CAD build for the part. Positions are in the model's coordinates, mm. A direction names the side the tool comes from. Round coordinates to 2 decimals unless told otherwise and drop trailing zeros. Order: outer loops, then holes, each group sorted by start corner. A loop starts at its lowest first (then second) coordinate and runs counter-clockwise, first axis right, second up.
Autodesk Inventor part; units mm, degrees
ref_plane "YZ Plane" through (0, 0, 0) normal (1, 0, 0) x (0, 1, 0)
ref_plane "XZ Plane" through (0, 0, 0) normal (0, 1, 0) x (-1, 0, 0)
ref_plane "XY Plane" through (0, 0, 0) normal (0, 0, 1) x (1, 0, 0)
sketch "Sketch1" plane through (0, 0, 0) normal (0, 0, 1) x (1, 0, 0)
  line L0 (-24.7628, 24.1619) -> (95.2372, 24.1619)
  line L1 (95.2372, 24.1619) -> (95.2372, -75.8381)
  line L2 (95.2372, -75.8381) -> (-24.7628, -75.8381)
  line L3 (-24.7628, -75.8381) -> (-24.7628, 24.1619)
  point P0 (0, 0)
  dimension "d0" = 120
  dimension "d1" = 100
extrude "Extrusion1" add sketch "Sketch1" along normal blind 80
sketch "Sketch2" plane through (-24.7628, -75.8381, 0) normal (-1, 0, 0) x (0, 0, 1)
  line L0 (0, 0) -> (80, 0)
  line L1 (4.914, 93.7072) -> (77, 93.7072)
  line L2 (77, 93.7072) -> (77, 0)
  line L3 (77, 0) -> (4.914, 0)
  line L4 (4.914, 0) -> (4.914, 93.7072)
  line L5 (80, 100) -> (80, 0)
  line L6 (0, 100) -> (0, 0)
  point P0 (0, 75.8381)
  point P1 (4.914, 0)
  dimension "d6" = 3
  dimension "d108" = 4.914
extrude "Extrusion2" cut sketch "Sketch2" against normal blind 60
sketch "Sketch3" plane through (-24.7628, 24.1619, 0) normal (0, 1, 0) x (1, 0, 0)
  line L0 (0, 0) -> (0, -4.914)
  line L1 (0, 0) -> (0, -31.38)
  circle A0 centre (26.718, -35) radius 11
  line L2 (120, 0) -> (0, 0)
  point P0 (24.7628, 0)
  dimension "d7" = 31.38
  dimension "d9" = 22
  dimension "d109" = 35
extrude "Extrusion3" cut sketch "Sketch3" against normal blind 80
sketch "Sketch8" plane through (0, 0, 0) normal (0, 0, -1) x (-1, 0, 0)
  line L0 (-95.2372, 24.1619) -> (24.7628, 24.1619)
  line L1 (-1.9784, 24.1619) -> (-38.1484, 24.1619)
  circle A0 centre (-1.7434, -26.1683) radius 3.5
  circle A1 centre (-10.4934, -46.1683) radius 1.575
  circle A2 centre (7.0066, -46.1683) radius 1.575
  line L2 (7.0066, -46.1683) -> (-10.4934, -46.1683)
  line L3 (-1.7434, -26.1683) -> (-1.7434, -46.1683)
  point P0 (0, 0)
  point P1 (-4.8068, -28.0128)
  dimension "d26" = 36.17
  dimension "d143" = 3.15
  dimension "d144" = 3.15
  dimension "d145" = 20
sketch "Sketch9" plane through (0, 0, 80) normal (0, 0, 1) x (1, 0, 0)
  line L0 (95.2372, 24.1619) -> (-24.7628, 24.1619)
  line L1 (41.408, 24.1619) -> (95.2372, 24.1619)
  line L2 (95.2372, 24.1619) -> (95.2372, -75.6591)
  line L3 (95.2372, -75.6591) -> (41.408, -75.6591)
  line L4 (41.408, -75.6591) -> (41.408, 24.1619)
  point P0 (0, 0)
extrude "Extrusion8" cut sketch "Sketch9" against normal blind 82.75
sketch "Sketch11" plane through (41.408, -75.6591, 80) normal (0, 1, 0) x (1, 0, 0)
  line L0 (0, 0) -> (-66.1708, 0)
  line L1 (-66.1708, 80) -> (53.8292, 80)
  line L2 (0, 0) -> (53.8292, 0)
  line L3 (53.8292, 0) -> (53.8292, 80)
  line L4 (53.8292, 80) -> (0, 80)
  line L5 (0, 80) -> (0, 0)
  point P0 (-41.408, 80)
extrude "Extrusion9" cut sketch "Sketch11" against normal blind 82.75
sketch "Sketch16" plane through (-24.7628, -75.8381, 77) normal (0, -1, 0) x (1, 0, 0)
  line L0 (0, -72.086) -> (0, 0)
  line L1 (0, 0) -> (60, 0)
  line L2 (0, -72.086) -> (60, -72.086)
  line L3 (60, -72.086) -> (60, 0)
  line L4 (60, 0) -> (0, 0)
  line L5 (0, 0) -> (0, -72.086)
  circle A0 centre (26.718, -42) radius 11
  circle A1 centre (26.718, -42) radius 5
  point P0 (24.7628, -77)
extrude "Extrusion14" add sketch "Sketch16" against normal blind 10 contours L0 L1 L3 L2
ref_plane "Work Plane1" through (-34.7628, -75.8381, 80) normal (-1, 0, 0) x (0, 0, 1)
sketch "Sketch24" plane through (-34.7628, -75.8381, 80) normal (-1, 0, 0) x (0, 0, 1)
  line L0 (-131.9676, 100) -> (-77.9351, 100)
  line L1 (-77.9351, 100) -> (-77.9351, -1.253)
  line L2 (-77.9351, -1.253) -> (-131.9676, -1.253)
  line L3 (-131.9676, -1.253) -> (-131.9676, 100)
  point P0 (-80, 75.8381)
extrude "Extrusion19" cut sketch "Sketch24" against normal blind 103.25
sketch "Sketch27" plane through (0, 0, 80) normal (0, 0, 1) x (1, 0, 0)
  line L0 (-24.7628, -75.8381) -> (41.408, -75.8381)
  circle A0 centre (15.3226, -32.8381) radius 1.5
  line L1 (15.3226, -32.8381) -> (1.3226, -32.8381)
  line L2 (15.3226, -35.3779) -> (15.3226, -32.8381)
  circle A1 centre (15.3226, -27.8381) radius 1.5
  circle A2 centre (1.3226, -32.8381) radius 1.5
  circle A3 centre (1.3226, -27.8381) radius 1.5
  line L3 (41.408, 24.1619) -> (-24.7628, 24.1619)
  point P0 (0, 0)
  dimension "d125" = 5
  dimension "d128" = 14
  dimension "d169" = 52
extrude "Extrusion22" cut sketch "Sketch27" against normal blind 20
extrude "Extrusion24" cut sketch "Sketch8" against normal blind 10
sketch "Sketch28" plane through (41.408, 24.1619, 2.0649) normal (0, 0, -1) x (-1, 0, 0)
  line L0 (0, -100) -> (0, 0)
  line L1 (66.1708, -90) -> (66.1708, -6.2928)
  line L2 (0, 0) -> (66.1708, 0)
  line L3 (66.1708, 0) -> (66.1708, -12.3951)
  line L4 (66.1708, -12.3951) -> (0, -12.3951)
  line L5 (0, -12.3951) -> (0, 0)
  point P0 (41.408, -24.1619)
  point P1 (0, -12.3951)
extrude "Extrusion25" add sketch "Sketch28" along normal blind 80
sketch "Sketch29" plane through (-24.7628, 11.7668, 2.0649) normal (0, -1, 0) x (1, 0, 0)
  line L0 (66.1708, -80) -> (0, -80)
  line L1 (66.1708, -80) -> (66.1708, -78.32)
  line L2 (66.1708, 0) -> (66.1708, -80)
  circle A0 centre (56.4908, -78.32) radius 0.75
  line L3 (56.4908, -78.32) -> (13.4908, -78.32)
  line L4 (56.4908, -61.93) -> (56.4908, -78.32)
  circle A1 centre (13.4908, -78.32) radius 0.75
  circle A2 centre (56.4908, -60.32) radius 0.75
  circle A3 centre (13.4908, -60.32) radius 0.75
  point P0 (24.7628, -2.0649)
  dimension "d150" = 1.5
  dimension "d155" = 43
  dimension "d158" = 18
  dimension "d163" = 18
extrude "Extrusion26" cut sketch "Sketch29" against normal blind 10
sketch "Sketch30" plane through (-24.7628, 11.7668, 2.0649) normal (0, -1, 0) x (1, 0, 0)
  circle A0 centre (56.4908, -78.32) radius 0.75
  line L0 (0, -80) -> (66.1708, -80)
  line L1 (43.4258, -80) -> (25.7382, -80)
  line L2 (25.7382, -80) -> (25.7382, -75)
  line L3 (25.7382, -75) -> (43.4258, -75)
  line L4 (43.4258, -75) -> (43.4258, -80)
  point P0 (24.7628, -2.0649)
  point P1 (25.7382, -80)
  point P2 (43.4258, -80)
  dimension "d165" = 5
  dimension "d168" = 13.065
extrude "Extrusion27" cut sketch "Sketch30" against normal blind 6 contours L2 L3 L4 L0
properties part number "Gearbox"
1. Tool access for faces 5 (the face through (10, 15, -72.935)), 6 (the face through (8, -31, 2.065)), 7 (the face through (-7.733, -47.566, 3.47)), 8 (the face through (5, 17.869, 48)): list every direction of +Z, -Z, +X, -X, +Y, -Y with a clear straight run to the whole face (end or side of a thin tool).
2. Cut at D-D, the plane z = -29.5. Write the cut outline in (x, y).
3. Cut at A-A, the plane z = 35. Write the cut outline in (x, y), and give its area (3 significant figures).
4. Cut at C-C, the plane z = 17.5. Write the cut outline in (x, y), and give its area (3 significant figures).
5. Mould opens along Y. For faces 1 (the face through (9, 18, -77.935)), 2 (the face through (-1.49, -27.51, 3.47)), 3 (the face through (0.997, -34.302, 78.521)), 4 (the face through (15, -75.838, 42)) say: released by +Y, released by -Y, zero draft, split by the parting line, or undercut.
6. Cut at B-B, the plane y = -38. Write the cut outline in (x, z).
7. Pin check, flat tips, straight feed: P1, Ø10, axis at y = -57, z = 63.5, coming from the -X side; P2, Ø4, axis at x = 15.32, y = -32.84, coming from the -Z side; P3, Ø1.5, axis at x = 14, z = -74.5, coming from the -Y side. Stop position of each tip, or through.
8. Drill centre lines: line 1 (Y direction, x = 1, z = 64); line 2 (Z direction, x = 27.5, y = -13); line 3 (Z direction, x = 22.5, y = 14.5). Where is each one in solid material? Low to high.
Outcome:
1. face 5: -Z, -Y
1. face 6: -Z, +X, -X, -Y
1. face 7: -Z
1. face 8: -X
2. outline: (-24.76, 11.77) - (41.41, 11.77) - (41.41, 24.16) - (-24.76, 24.16) - close
3. outline: (-24.76, -75.84) - (-9.04, -75.84) - (-9.04, -65.84) - (-24.76, -65.84) - close; (-24.76, 17.87) - (-9.04, 17.87) - (-9.04, 24.16) - (-24.76, 24.16) - close; (12.96, -75.84) - (41.41, -75.84) - (41.41, 24.16) - (12.96, 24.16) - (12.96, 17.87) - (35.24, 17.87) - (35.24, -65.84) - (12.96, -65.84) - close
3. area: 1,240 mm2
4. outline: (-24.76, -75.84) - (41.41, -75.84) - (41.41, 24.16) - (-24.76, 24.16) - (-24.76, 17.87) - (35.24, 17.87) - (35.24, -65.84) - (-24.76, -65.84) - close
4. area: 1,590 mm2
5. face 1: zero draft
5. face 2: undercut
5. face 3: undercut
5. face 4: released by -Y
6. outline: (-24.76, 2.06) - (41.41, 2.06) - (41.41, 80) - (-24.76, 80) - (-24.76, 77) - (35.24, 77) - (35.24, 4.91) - (-24.76, 4.91) - close
7. P1: stops at x = 35.24
7. P2: stops at z = 2.06
7. P3: stops at y = 17.77
8. line 1: y = -75.84 to -65.84, 17.87 to 24.16
8. line 2: z = 2.06 to 4.91, 77 to 80
8. line 3: z = -77.94 to 4.91, 77 to 80
